Build history of the part. All positions in model axes, mm. Face numbers are marked on the shaded views. A direction names the side the tool comes from. Coordinates: 2 decimals unless noted, no trailing zeros. Write each loop counter-clockwise with the first axis right and the second up, starting at its lowest first coordinate (ties: lowest second). Pieces come first, ordered by that corner, then holes.
Autodesk Inventor part; units mm, degrees
ref_plane "YZ Plane" through (0, 0, 0) normal (1, 0, 0) x (0, 1, 0)
ref_plane "XZ Plane" through (0, 0, 0) normal (0, 1, 0) x (-1, 0, 0)
ref_plane "XY Plane" through (0, 0, 0) normal (0, 0, 1) x (1, 0, 0)
sketch "Sketch1" plane through (0, 0, 0) normal (0, 0, 1) x (1, 0, 0)
  circle A0 centre (0, 0) radius 2.5
  dimension "d0" = 5
extrude "Extrusion1" add sketch "Sketch1" along normal blind 50
sketch "Sketch2" plane through (0, 0, 50) normal (0, 0, 1) x (1, 0, 0)
  circle A0 centre (0, 0) radius 3.5
  dimension "d3" = 7
extrude "Extrusion2" add sketch "Sketch2" along normal blind 20
sketch "Sketch3" plane through (0, 0, 70) normal (0, 0, 1) x (1, 0, 0)
  point P0 (0, 0)
  point P1 (0, 0)
hole "Hole1" at (0, 0, 70) direction (0, 0, -1) diameter 5.3 depth 15
equation "\"fitTol\" = 0.3"
properties part number "RCPlaneConnectorTest"
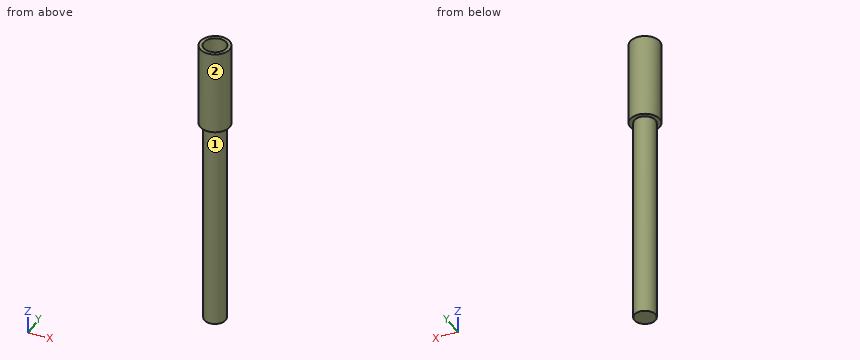
1. Flat gauge pins, fed straight in: pin 1 (1.5 mm diameter, centred on x = 0.5, y = 1, fed in from -Z); pin 2 (4 mm diameter, centred on x = 0.5, z = 34.5, fed in from +Y); pin 3 (1 mm diameter, centred on x = -1, z = 55.5, fed in from +Y). Where does each tip first touch, or does it go through?
Computed values:
pin 1: stops at z = 0
pin 2: stops at y = 2.5
pin 3: stops at y = 3.46
2. 3-axis set-ups, long thin cutter, end or side, ignore diameter. For the marked faces 1 and 2: which of +Z, -Z, +X, -X, +Y, -Y reach the whole face in a straight line?
Computed values:
face 1: -Z
face 2: +Z, -Z
3. Saw through at C-C on z = 62. List the corners of the cut face in (x, y), plus the area to 3 significant figures.
Computed values:
outline: circle Ø7 at (0, 0); hole circle Ø5.3 at (0, 0)
area: 16.4 mm2
4. Saw through at D-D on z = 52. List the corners of the cut face in (x, y).
Computed values:
outline: circle Ø7 at (0, 0)
5. Probe line 1 along Y through (x, z) = (0, 62.75); line 2 along Z through (x, y) = (2.25, 0.25); line 3 along Z through (x, y) = (1.5, 3). List the from-to ranges inside material, lowest first.
Computed values:
line 1: y = -3.5 to -2.65, 2.65 to 3.5
line 2: z = 0 to 55
line 3: z = 50 to 70
6. Saw through at A-A on y = 0. List the corners of the cut face in (x, z), plus the area to 4 significant figures.
Computed values:
outline: (-3.5, 50) - (-2.5, 50) - (-2.5, 0) - (2.5, 0) - (2.5, 50) - (3.5, 50) - (3.5, 70) - (2.65, 70) - (2.65, 55) - (-2.65, 55) - (-2.65, 70) - (-3.5, 70) - close
area: 310.5 mm2
